Build history of the part. All positions in model axes, mm. A direction names the side the tool comes from. Give positions to 0.01 mm unless a question says otherwise; leave off trailing zeros. Loops run counter-clockwise (first coordinate to the right, second up) from the corner with the lowest first, then second, coordinate; pieces in that order, holes last.
1) Wall check: line 1 (X direction, y = 241, z = 5.5); line 2 (Z direction, x = 41.5, y = 273.5); line 3 (Z direction, x = 11.5, y = 252.5). Give the ranges that are in metal, low to high.
2) Band-saw the part on A-A on z = 22. List the corners of the cut face in (x, y).
3) Band-saw the part on B-B on y = 222. List the corners of the cut face in (x, z), then the cut area to 3 significant figures.
4) Two-plate mould, pull along X, no slides. Class faces 3 (the cylindrical face through (69.37, 202.13, -1.51)), 4 (the flat face through (40, 208, 4)), 5 (the flat face through (40, 410, 2)), 6 (the cylindrical face through (10.63, 207.87, -1.51)): +X half, -X half, draft (parallel to the pull), parting line (faces both ways), or undercut.
5) 3-axis set-ups, long thin cutter, end or side, ignore diameter. For faces 1 (the flat face through (64, 202, 33)), 2 (the flat face through (40, 208, -4)): which of +Z, -Z, +X, -X, +Y, -Y reach the whole face in a straight line?
6) Band-saw the part on C-C on x = 35.5. List the corners of the cut face in (y, z), then the cut area to 3 significant figures.
```python
from build123d import *

# Parameters (mm, degrees)
SM_START                           = -4
SM_BASE_FLANGE_1_OUTLINE_W         = 64
SM_BASE_FLANGE_1_OUTLINE_H         = 410
SM_BASE_FLANGE_1_DEPTH             = 8
SM_EDGE_FLANGE_1_STRIP_W           = 33.4732
SM_EDGE_FLANGE_1_STRIP_H           = 8
SM_EDGE_FLANGE_1_STRIP_CUT_DEPTH   = 410
SM_EDGE_FLANGE_1_STRIP_2_W         = 33.4732
SM_EDGE_FLANGE_1_STRIP_2_H         = 8
SM_EDGE_FLANGE_1_STRIP_CUT_2_DEPTH = 410
SM_EDGE_FLANGE_1_DEPTH             = 410
SM_EDGE_FLANGE_1_BEND_DEPTH        = 410


# Read off the part's stored shape, not the designer's step: 基体-法兰1
# Sheet-metal steps are written as plain solids
with BuildPart() as part:
    # 基体-法兰1 outline → 基体-法兰1 (new body)
    with BuildSketch(Plane.XY.offset(SM_START)):
        with Locations((40, 205)):
            Rectangle(SM_BASE_FLANGE_1_OUTLINE_W, SM_BASE_FLANGE_1_OUTLINE_H)
    extrude(amount=SM_BASE_FLANGE_1_DEPTH)

    # 边线-法兰1 strip (across the edge) → 边线-法兰1 strip cut (cut)
    with BuildSketch(Plane(origin=(8, 410, 4), x_dir=(1, 0, 0), z_dir=(0, -1, 0))):
        with Locations((-8, -4)):
            Rectangle(SM_EDGE_FLANGE_1_STRIP_W, SM_EDGE_FLANGE_1_STRIP_H)
    extrude(amount=SM_EDGE_FLANGE_1_STRIP_CUT_DEPTH, mode=Mode.SUBTRACT)

    # 边线-法兰1 strip 2 (across the edge) → 边线-法兰1 strip cut 2 (cut)
    with BuildSketch(Plane(origin=(72, 0, 4), x_dir=(-1, 0, 0), z_dir=(0, 1, 0))):
        with Locations((-8, -4)):
            Rectangle(SM_EDGE_FLANGE_1_STRIP_2_W, SM_EDGE_FLANGE_1_STRIP_2_H)
    extrude(amount=SM_EDGE_FLANGE_1_STRIP_CUT_2_DEPTH, mode=Mode.SUBTRACT)

    # 边线-法兰1 section (across the edge) → 边线-法兰1 (add)
    with BuildSketch(Plane(origin=(8, 410, 4), x_dir=(1, 0, 0), z_dir=(0, -1, 0))):
        with BuildLine():
            Line((0, 0.7366), (0, 56))
            Line((0, 56), (8, 56))
            Line((8, 56), (8, 0.7366))
            ThreePointArc((8, 0.7366), (8.215745145, 0.215745145), (8.7366, 0))
            Line((8.7366, 0), (8.7366, -8))
            ThreePointArc((8.7366, -8), (2.558890895, -5.441109105), (0, 0.7366))
        make_face()
    extrude(amount=SM_EDGE_FLANGE_1_DEPTH)

    # 边线-法兰1 section 2 (across the edge) → 边线-法兰1 bend (add)
    with BuildSketch(Plane(origin=(72, 0, 4), x_dir=(-1, 0, 0), z_dir=(0, 1, 0))):
        with BuildLine():
            Line((0, 0.7366), (0, 56))
            Line((0, 56), (8, 56))
            Line((8, 56), (8, 0.7366))
            ThreePointArc((8, 0.7366), (8.215745145, 0.215745145), (8.7366, 0))
            Line((8.7366, 0), (8.7366, -8))
            ThreePointArc((8.7366, -8), (2.558890895, -5.441109105), (0, 0.7366))
        make_face()
    extrude(amount=SM_EDGE_FLANGE_1_BEND_DEPTH)


solid = part.part
```
Findings below:
1. line 1: x = 8 to 16, 64 to 72
1. line 2: z = -4 to 4
1. line 3: z = -2.26 to 60
2. outline: (8, 0) - (16, 0) - (16, 410) - (8, 410) - close; (64, 0) - (72, 0) - (72, 410) - (64, 410) - close
3. outline: (8, 4.74) arc R8.74 ccw to (16.74, -4) - (63.26, -4) arc R8.74 ccw to (72, 4.74) - (72, 60) - (64, 60) - (64, 4.74) arc R0.74 cw to (63.26, 4) - (16.74, 4) arc R0.74 cw to (16, 4.74) - (16, 60) - (8, 60) - close
3. area: 1,380 mm2
4. face 3: +X half
4. face 4: undercut
4. face 5: draft
4. face 6: -X half
5. face 1: +Z, +Y, -Y
5. face 2: -Z, +X, -X, +Y, -Y
6. outline: (0, -4) - (410, -4) - (410, 4) - (0, 4) - close
6. area: 3,280 mm2
